Geometry check sheet. Reference: the model listing, model coordinates, mm. Face numbers are marked on the shaded views. A direction names the side the tool comes from. Round coordinates to 2 decimals unless told otherwise and drop trailing zeros. Write each loop counter-clockwise with the first axis right and the second up, starting at its lowest first coordinate (ties: lowest second). Pieces come first, ordered by that corner, then holes. Notation, with made-up numbers: (-39.75, -14) - (14.25, -14) arc R18 ccw to (14.25, 19) - close; hole circle Ø1 at (17, 7). An arc over 180 degrees is marked (long way). Return JSON: item names as keys, results as strings.
```python
from build123d import *

# Parameters (mm, degrees)
BOSS_EXTRUDE1_DEPTH                     = 5
SKETCH4_W                               = 15
SKETCH4_H                               = 14
BOSS_EXTRUDE2_DEPTH                     = 5
CBORE_FOR_M6_HEX_HEAD_BOLT1_D           = 6.647
CBORE_FOR_M6_HEX_HEAD_BOLT1_DEPTH       = 10
CBORE_FOR_M6_HEX_HEAD_BOLT1_CBORE_D     = 9
CBORE_FOR_M6_HEX_HEAD_BOLT1_CBORE_DEPTH = 2
CBORE_FOR_M6_HEX_HEAD_BOLT1_TIP         = 1.996960267
FILLET1_R                               = 1
FILLET2_R                               = 4
TAP_DRILL_FOR_M3X0_5_TAP1_D             = 2.5


with BuildPart() as part:
    # Sketch1 → Boss-Extrude1 (new body)
    with BuildSketch(Plane(origin=(0, 0, 0), x_dir=(-1, 0, 0), z_dir=(0, 0, -1))):
        with BuildLine():
            Line((27.500000074, -16.263075607), (27.500000074, 0))
            Line((27.500000074, 0), (-27.5, 0))
            Line((-27.5, 0), (-27.5, -16.2630756))
            ThreePointArc((-27.5, -16.2630756), (3.7e-08, -15), (27.500000074, -16.263075607))
        make_face()
    extrude(amount=-BOSS_EXTRUDE1_DEPTH)

    # Sketch4 → Boss-Extrude2 (add)
    with BuildSketch(Plane.XY.offset(5)):
        with Locations((0, -7)):
            Rectangle(SKETCH4_W, SKETCH4_H)
    extrude(amount=BOSS_EXTRUDE2_DEPTH)

    # CBORE for M6 Hex Head Bolt1
    with Locations(Plane(origin=(0, 0, 0), x_dir=(1, 0, 0), z_dir=(0, 1, 0))):
        with Locations((0, -5)):
            CounterBoreHole(CBORE_FOR_M6_HEX_HEAD_BOLT1_D / 2, CBORE_FOR_M6_HEX_HEAD_BOLT1_CBORE_D / 2, CBORE_FOR_M6_HEX_HEAD_BOLT1_CBORE_DEPTH, depth=CBORE_FOR_M6_HEX_HEAD_BOLT1_DEPTH)
            with Locations((0, 0, -(CBORE_FOR_M6_HEX_HEAD_BOLT1_DEPTH + CBORE_FOR_M6_HEX_HEAD_BOLT1_TIP / 2))):  # 118° drill point
                Cone(0, CBORE_FOR_M6_HEX_HEAD_BOLT1_D / 2, CBORE_FOR_M6_HEX_HEAD_BOLT1_TIP, mode=Mode.SUBTRACT)

    # Fillet1
    fillet1_edges = [part.edges().sort_by_distance(p)[0] for p in [
        (27.5, 0, 2.5),
        (-27.500000074, 0, 2.5),
    ]]
    fillet(fillet1_edges, radius=FILLET1_R)

    # Fillet2
    fillet2_edges = [part.edges().sort_by_distance(p)[0] for p in [
        (7.5, -14, 7.5),
        (7.5, -7, 10),
        (-7.5, -14, 7.5),
        (0, -14, 10),
        (-7.5, -7, 10),
    ]]
    fillet(fillet2_edges, radius=FILLET2_R)

    # Tap Drill for M3x0.5 Tap1 (through all)
    with Locations(Plane(origin=(-10.5, -2.5, 5), x_dir=(1, 0, 0), z_dir=(0, 0, 1))):
        with Locations((0, 0), (21, 0)):
            Hole(TAP_DRILL_FOR_M3X0_5_TAP1_D / 2)


solid = part.part
```
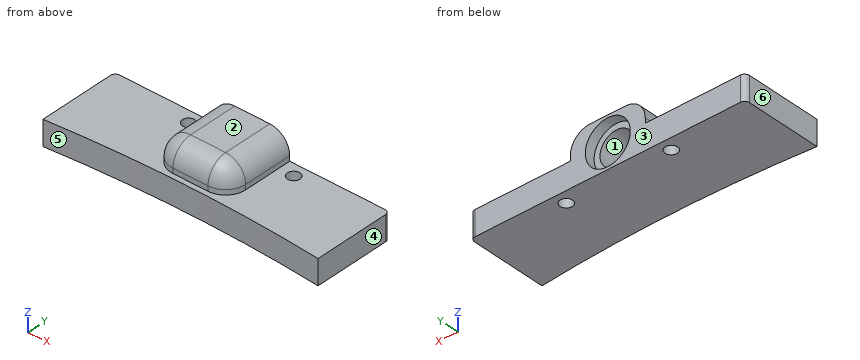
(1) Gauge pin test, flat ends, axial feed: pin 1 (5 mm diameter, centred on x = -7.5, y = -2.5, fed in from +Z); pin 2 (3 mm diameter, centred on x = -15.5, z = 3.5, fed in from -Y); pin 3 (8 mm diameter, centred on x = -12, y = -6, fed in from +Z). Record the tip position at first contact, or that the pin passes through.
Response values:
{"pin 1": "stops at z = 9.71", "pin 2": "stops at y = -15.48", "pin 3": "stops at z = 5"}
(2) Section check D-D, the plane y = -13. Enter the section's corners in (x, z), plus the area to 3 significant figures.
Response values:
{"outline": "(-27.5, 0) - (27.5, 0) - (27.5, 5) - (6.15, 5) - (6.15, 6) arc R2.65 ccw to (3.5, 8.65) - (-3.5, 8.65) arc R2.65 ccw to (-6.15, 6) - (-6.15, 5) - (-27.5, 5) - close", "area": "317 mm^2"}
(3) Section check B-B, the plane y = -8.25. Enter the section's corners in (x, z).
Response values:
{"outline": "(-27.5, 0) - (27.5, 0) - (27.5, 5) - (7.5, 5) - (7.5, 6) arc R4 ccw to (3.5, 10) - (-3.5, 10) arc R4 ccw to (-7.5, 6) - (-7.5, 5) - (-27.5, 5) - close; hole circle Ø6.65 at (0, 5)"}
(4) Access from +Z, -Z, +X, -X, +Y, -Y to the whole of each face (thin tool, end or side, straight path). Record for the marked faces 1 and 2.
Response values:
{"face 1": "+Y", "face 2": "+Z, +X, -X, +Y, -Y"}
(5) Material ranges on line 1 along Z through (x, y) = (0, -7.25); line 2 along Z through (x, y) = (-23, -2.25); line 3 along Z through (x, y) = (-2.5, -1.75), recorded low to high. Write a range as [from, to].
Response values:
{"line 1": "z = [0, 1.68], [8.32, 10]", "line 2": "z = [0, 5]", "line 3": "z = [0, 1.26], [8.74, 10]"}
(6) Release check for a two-part mould opening along X. For the marked faces 3, 4, 5 and 6 record: pulls with the +X half, pulls with the -X half, needs draft (parallel to the pull), parting line crosses it, or undercut.
Response values:
{"face 3": "needs draft", "face 4": "pulls with the +X half", "face 5": "undercut", "face 6": "pulls with the -X half"}
(7) Section check C-C, the plane x = 10.5. Enter the section's corners in (y, z).
Response values:
{"outline": "(-15.18, 0) - (-3.75, 0) - (-3.75, 5) - (-15.18, 5) - close; (-1.25, 0) - (0, 0) - (0, 5) - (-1.25, 5) - close"}
(8) Section check A-A, the plane y = -2.5. Enter the section's corners in (x, z), plus the area to 3 significant figures.
Response values:
{"outline": "(-27.5, 0) - (-11.75, 0) - (-11.75, 5) - (-27.5, 5) - close; (-9.25, 0) - (9.25, 0) - (9.25, 5) - (7.5, 5) - (7.5, 6) arc R4 ccw to (3.5, 10) - (-3.5, 10) arc R4 ccw to (-7.5, 6) - (-7.5, 5) - (-9.25, 5) - close; (11.75, 0) - (27.5, 0) - (27.5, 5) - (11.75, 5) - close; hole circle Ø6.65 at (0, 5)", "area": "283 mm^2"}
